Part model, mm, in its own coordinate system. A direction names the side the tool comes from. Give positions to 0.01 mm unless a question says otherwise; leave off trailing zeros. Order: outer loops, then holes, each group sorted by start corner. A loop starts at its lowest first (then second) coordinate and runs counter-clockwise, first axis right, second up. Notation, with made-up numbers: (53.5, 48.25) - (66.5, 48.25) arc R15 ccw to (66.5, 53.25) - close; hole circle Ø11 at (66.25, -23.5). An arc over 180 degrees is marked (long way). Use a Markdown table: item, result. Add a question column.
from build123d import *

# Parameters (mm, degrees)
BOSS_EXTRUDE1_DEPTH = 24
BOSS_EXTRUDE1_DRAFT = -8
SCALE1_SCALE        = 4
SKETCH3_R           = 45
CUT_EXTRUDE1_DEPTH  = 88
SKETCH4_R           = 29.815
CUT_EXTRUDE2_DEPTH  = 96


with BuildPart() as part:
    # Sketch1 → Boss-Extrude1 (with draft: the straight prism first)
    with BuildSketch(Plane.XY):
        Polygon((-53.266019417, 16.909847434), (-59.184466019, -7.891262136), (-20.573647712, -7.891262136), (-23.110124827, 14.65520111), (-36.919833564, 23.391955617), align=None)
    extrude(amount=BOSS_EXTRUDE1_DEPTH)
    # Boss-Extrude1: the draft: its side faces are tilted about the plane it starts from
    boss_extrude1_sides = [part.faces().sort_by_distance(p)[0] for p in [
        (-56.225242718, 4.509292649, 12),
        (-39.879056865, -7.891262136, 12),
        (-21.841886269, 3.381969487, 12),
        (-30.014979196, 19.023578363, 12),
        (-45.092926491, 20.150901526, 12),
    ]]
    draft(boss_extrude1_sides, Plane.XY, BOSS_EXTRUDE1_DRAFT)


with BuildPart() as part_1:
    # Scale1: scaled about (-39.217709301, 5.154172018, 12.784931537)
    add(part.part.scale(SCALE1_SCALE).moved(Location((117.653127903, -15.462516054, -38.354794611))))

    # Sketch3 → Cut-Extrude1 (cut)
    with BuildSketch(Plane(origin=(0, 138, 0), x_dir=(1, 0, 0), z_dir=(0, 1, 0))):
        with Locations(Location((-29.321171046, -9.645205389, 0), (0, 0, 270))):
            Circle(SKETCH3_R)
    extrude(amount=-CUT_EXTRUDE1_DEPTH, mode=Mode.SUBTRACT)

    # Sketch4 → Cut-Extrude2 (cut)
    with BuildSketch(Plane.XY.offset(57.645205389)):
        with Locations((-38.993157732, 0.806531709)):
            Circle(SKETCH4_R)
    extrude(amount=-CUT_EXTRUDE2_DEPTH, mode=Mode.SUBTRACT)


solid = part_1.part
1. Tool access for faces 1 (the face through (-26, 30, -38.355)), 2 (the face through (-69.244, 62.162, 30.41)): list every direction of +Z, -Z, +X, -X, +Y, -Y with a clear straight run to the whole face (end or side of a thin tool).
2. Cut at D-D (y = 56.5). Write the cut outline in (x, z), plus the area to 3 significant figures.
3. Drill centre lines: probe 1 along X at (y, z) = (19, -31); probe 2 along X at (y, z) = (8, 33); probe 3 along Y at (x, z) = (-14, 52.5). Where is each one in solid material? Low to high. Write a range as [from, to].
4. Pin check, flat tips, straight feed: P1, Ø4, axis at y = -28.5, z = 16.5, coming from the +X side; P2, Ø4, axis at y = 8.5, z = -6.5, coming from the +X side; P3, Ø10, axis at x = -26.5, z = 40, coming from the +Y side. Stop position of each tip, or through.
5. Cut at A-A (x = -13.5). Write the cut outline in (y, z).
6. Cut at C-C (z = -2). Write the cut outline in (x, y) (3 decimals).
7. Cut at B-B (y = -13.5). Write the cut outline in (x, z).
8. Mould opens along Z. For faces 3 (the face through (37.465, -6.256, 8.973)), 4 (the face through (-10.555, 9.762, 10.317)), 5 (the face through (-29, 50, 9)) say: released by +Z, released by -Z, zero draft, split by the parting line, or undercut.
Responses:
| question | item | result |
|---|---|---|
| 1 | face 1 | -Z, +X, -X, +Y, -Y |
| 1 | face 2 | +Y |
| 2 | outline | (-108.25, 57.65) - (-100.4, 3.33) - (-84.51, -38.35) - (4.12, -38.35) - (12.15, -7.82) arc R45 cw (long way) to (15.38, 4.46) - (29.36, 57.65) - close |
| 2 | area | 4,770 mm² |
| 3 | probe 1 | x = [-104.39, -62.61], [-15.37, 28.97] |
| 3 | probe 2 | x = [-116.26, -67.93], [-10.06, 39.26] |
| 3 | probe 3 | y = [-59.8, -15.45], [17.06, 83.08] |
| 4 | P1 | stops at x = 41.39 |
| 4 | P2 | stops at x = 33.98 |
| 4 | P3 | stops at y = 50 |
| 5 | outline | (-60.52, 57.65) - (-47.03, -38.35) - (-14.65, -38.35) - (-14.65, 57.65) - close; (16.27, -38.35) - (67.65, -38.35) - (68.63, -32.48) - (50, -32.48) - (50, 51.77) - (82.64, 51.77) - (83.62, 57.65) - (16.27, 57.65) - close |
| 6 | outline | (-125.557, -52.137) - (41.075, -52.137) - (30.016, 46.165) - (14.146, 56.206) - (14.146, 50) - (-72.788, 50) - (-72.788, 66.644) - (-99.764, 55.947) - close; hole circle Ø59.63 at (-38.993, 0.807) |
| 7 | outline | (-124.95, 57.65) - (-111.08, -38.35) - (-65.15, -38.35) - (-65.15, 57.65) - close; (-12.83, -38.35) - (31.59, -38.35) - (45.16, 57.65) - (-12.83, 57.65) - close |
| 8 | face 3 | released by -Z |
| 8 | face 4 | zero draft |
| 8 | face 5 | undercut |
